from build123d import *

# Parameters (mm, degrees)
BOSS_EXTRUDE1_DEPTH     = 24.209375
CUT_EXTRUDE1_DEPTH      = 65.637036854
CUT_EXTRUDE2_DEPTH      = 65.637036854
SKETCH4_R               = 3.175
CUT_EXTRUDE3_DEPTH      = 65.637036854
SKETCH5_W               = 7.14375
SKETCH5_H               = 12.7
SKETCH5_W_2             = 10.715625
SKETCH5_H_2             = 28.575
CUT_EXTRUDE4_DEPTH      = 65.637036854
CUT_EXTRUDE4_DEPTH_BACK = 65.637036854
SKETCH6_R               = 6.35
SKETCH6_R_2             = 3.175
BOSS_EXTRUDE2_DEPTH     = 3.175
SKETCH7_R               = 6.35
SKETCH7_R_2             = 3.175
BOSS_EXTRUDE4_DEPTH     = 3.175


with BuildPart() as part:
    # Sketch1 → Boss-Extrude1 (new body)
    with BuildSketch(Plane.XY):
        Polygon((-11.90625, 0), (11.90625, 0), (11.90625, -25.4), (11.90625, -58.7375), (-11.90625, -58.7375), (-11.90625, -25.4), align=None)
    extrude(amount=BOSS_EXTRUDE1_DEPTH)

    # Sketch2 → Cut-Extrude1 (cut, through all)
    with BuildSketch(Plane.XZ.offset(58.7375)):
        Polygon((-11.90625, 24.209375), (-11.90625, 7.540625), (-6.35, 24.209375), align=None)
        Polygon((11.90625, 24.209375), (6.35, 24.209375), (11.90625, 7.540625), align=None)
    extrude(amount=-CUT_EXTRUDE1_DEPTH, mode=Mode.SUBTRACT)

    # Sketch3 → Cut-Extrude2 (cut, through all)
    with BuildSketch(Plane.XY.offset(24.209375)):
        Polygon((-11.90625, -58.7375), (-6.35, -58.7375), (-6.35, -54.320108696), (-11.90625, -46.0375), align=None)
        Polygon((11.90625, -46.0375), (6.35, -54.320108696), (6.35, -58.7375), (11.90625, -58.7375), align=None)
        with BuildLine():
            Line((6.35, -54.320108696), (5.273356401, -55.925043253))
            ThreePointArc((5.273356401, -55.925043253), (2.988235294, -57.990441176), (0, -58.7375))
            Line((0, -58.7375), (6.35, -58.7375))
            Line((6.35, -58.7375), (6.35, -54.320108696))
        make_face()
        with BuildLine():
            Line((-6.35, -58.7375), (0, -58.7375))
            ThreePointArc((0, -58.7375), (-2.988235294, -57.990441176), (-5.273356401, -55.925043253))
            Line((-5.273356401, -55.925043253), (-6.35, -54.320108696))
            Line((-6.35, -54.320108696), (-6.35, -58.7375))
        make_face()
    extrude(amount=-CUT_EXTRUDE2_DEPTH, mode=Mode.SUBTRACT)

    # Sketch4 → Cut-Extrude3 (cut, through all)
    with BuildSketch(Plane.XY.offset(24.209375)):
        with Locations((0, -52.3875)):
            Circle(SKETCH4_R)
        with Locations((0, -36.5125)):
            Circle(SKETCH4_R)
    extrude(amount=-CUT_EXTRUDE3_DEPTH, mode=Mode.SUBTRACT)

    # Sketch5 → Cut-Extrude4 (cut, two sides)
    with BuildSketch(Plane(origin=(0, 0, 0), x_dir=(0, 0, -1), z_dir=(1, 0, 0))) as cut_extrude4_sk:
        with Locations((-17.4625, -52.3875)):
            Rectangle(SKETCH5_W, SKETCH5_H)
        with Locations((-17.4625, -36.5125)):
            Rectangle(SKETCH5_W, SKETCH5_H)
        with Locations((-5.3578125, -44.45)):
            Rectangle(SKETCH5_W_2, SKETCH5_H_2)
    extrude(amount=CUT_EXTRUDE4_DEPTH, mode=Mode.SUBTRACT)
    extrude(cut_extrude4_sk.sketch, amount=-CUT_EXTRUDE4_DEPTH_BACK, mode=Mode.SUBTRACT)

    # Sketch6 → Boss-Extrude2 (add)
    with BuildSketch(Plane.XY.offset(24.209375)):
        with Locations((0, -36.5125)):
            Circle(SKETCH6_R)
        with Locations((0, -36.5125)):
            Circle(SKETCH6_R_2, mode=Mode.SUBTRACT)
        with Locations((0, -52.3875)):
            Circle(SKETCH6_R)
        with Locations((0, -52.3875)):
            Circle(SKETCH6_R_2, mode=Mode.SUBTRACT)
    extrude(amount=BOSS_EXTRUDE2_DEPTH)

    # Sketch7 → Boss-Extrude4 (add)
    with BuildSketch(Plane(origin=(0, 0, 10.715625), x_dir=(-1, 0, 0), z_dir=(0, 0, -1))):
        with Locations(Location((0, -52.3875, 0), (0, 0, 213.855026128))):
            Circle(SKETCH7_R)
        with Locations(Location((0, -52.3875, 0), (0, 0, 180))):
            Circle(SKETCH7_R_2, mode=Mode.SUBTRACT)
        with BuildLine():
            Line((-3.175, -30.1625), (-3.175, -31.013238686))
            ThreePointArc((-3.175, -31.013238686), (0, -42.8625), (3.175, -31.013238686))
            Line((3.175, -31.013238686), (3.175, -30.1625))
            Line((3.175, -30.1625), (-3.175, -30.1625))
        make_face()
        with Locations(Location((0, -36.5125, 0), (0, 0, 180))):
            Circle(SKETCH7_R_2, mode=Mode.SUBTRACT)
    extrude(amount=BOSS_EXTRUDE4_DEPTH)


solid = part.part
Source: CAD feature listing. Evaluate the final solid. Frame: model axes, mm. A direction names the side the tool comes from. Round coordinates to 2 decimals unless told otherwise and drop trailing zeros. Loops run counter-clockwise (first coordinate to the right, second up) from the corner with the lowest first, then second, coordinate; pieces in that order, holes last. Notation, with made-up numbers: (61.25, 71.25) - (66.25, 71.25) arc R23 ccw to (66.25, 84.25) - close; hole circle Ø6 at (14.5, 74). An arc over 180 degrees is marked (long way). Write item = value, one per line. Start each with the question number.
Item 1: Reachability of faces 5 (the face through (-1.8, -39.4, 21.034)), 6 (the face through (-0.827, -30.217, 25.775)), 7 (the face through (0.23, -42.86, 9.15)) from +Z, -Z, +X, -X, +Y, -Y: full face, straight path, thin tool, end or side. Return the list, or none.
Item 2: Material intervals for line 1 (Y direction, x = 0, z = 9.1); line 2 (Y direction, x = 1, z = 11); line 3 (Z direction, x = 2.25, y = -41.5), sorted ascending.
Item 3: Section query A-A on z = 8.25. Count the separate pieces of the cut face and the enclosed holes in it, plus the area to 3 significant figures.
Item 4: Mould query, pull axis Z, two halves, no side actions, for faces 1 (the face through (0, -30.162, 18)), 2 (the face through (-3, -38, 27.384)), 3 (the face through (3.2, -51.1, 21.034)), 4 (the face through (-0.2, -43.2, 10.716)). Classes: released by +Z, released by -Z, zero draft, split by the parting line, or undercut.
Item 5: First-contact query: pin 1 Ø10 at (x, y) = (0.5, -37.5) entering from -Z; pin 2 Ø4 at (x, y) = (0, -52.39) entering from +Z; pin 3 Ø4 at (y, z) = (-19.5, 22) entering from +X; pin 4 Ø3 at (x, z) = (6, 15.5) entering from -Y. Flat tips, straight axial feed; report the tip coordinate or a pass-through.
Item 6: Section query D-D on x = 4. Output: boundary loops of the cut face in (y, z), plus the area to 3 significant figures.
Item 7: Section query C-C on y = -37.5. Output: boundary loops of the cut face in (x, z).
Item 8: Section query B-B on z = 19.5. Output: boundary loops of the cut face in (x, y), plus the area to 3 significant figures.
Results list:
q1.face_5 = +X, -X
q1.face_6 = +Z
q1.face_7 = -Z
q2.line_1 = -58.74 to -55.56, -49.21 to -46.04, -42.86 to -39.69, -33.34 to 0
q2.line_2 = -58.66 to -55.4, -49.37 to -39.53, -33.5 to 0
q2.line_3 = 7.54 to 13.89, 21.03 to 27.38
q3.separate_pieces = 2
q3.enclosed_holes = 2
q3.area = 896 mm²
q4.face_1 = undercut
q4.face_2 = released by +Z
q4.face_3 = undercut
q4.face_4 = released by -Z
q5.pin_1 = 7.54
q5.pin_2 = through
q5.pin_3 = 7.75
q5.pin_4 = -46.04
q6.outline = (-57.32, 7.54) - (-47.46, 7.54) - (-47.46, 10.72) - (-41.44, 10.72) - (-41.44, 7.54) - (-31.58, 7.54) - (-31.58, 10.72) - (-30.16, 10.72) - (-30.16, 0) - (0, 0) - (0, 24.21) - (-31.58, 24.21) - (-31.58, 27.38) - (-41.44, 27.38) - (-41.44, 24.21) - (-47.46, 24.21) - (-47.46, 27.38) - (-57.32, 27.38) - (-57.32, 21.03) - (-46.04, 21.03) - (-46.04, 13.89) - (-57.32, 13.89) - close; hole (-42.86, 13.89) - (-30.16, 13.89) - (-30.16, 21.03) - (-42.86, 21.03) - close
q6.area = 1,050 mm²
q7.outline = (-10.85, 10.72) - (-6.27, 10.72) - (-6.27, 7.54) - (-3.02, 7.54) - (-3.02, 13.89) - (-9.79, 13.89) - close; (-7.41, 21.03) - (-3.02, 21.03) - (-3.02, 27.38) - (-6.27, 27.38) - (-6.27, 24.21) - (-6.35, 24.21) - close; (3.02, 7.54) - (6.27, 7.54) - (6.27, 10.72) - (10.85, 10.72) - (9.79, 13.89) - (3.02, 13.89) - close; (3.02, 21.03) - (7.41, 21.03) - (6.35, 24.21) - (6.27, 24.21) - (6.27, 27.38) - (3.02, 27.38) - close
q8.outline = (-7.92, -46.04) - (7.92, -46.04) - (7.92, -42.86) - (-7.92, -42.86) - close; (-7.92, -30.16) - (7.92, -30.16) - (7.92, 0) - (-7.92, 0) - close
q8.area = 528 mm²
